Geometry: final body of the model. Coordinates: model frame, mm. Give positions to 0.01 mm unless a question says otherwise; leave off trailing zeros. Write each loop counter-clockwise with the first axis right and the second up, starting at its lowest first coordinate (ties: lowest second). Pieces come first, ordered by that corner, then holes.
Autodesk Inventor part; units mm, degrees
ref_plane "YZ Plane" through (0, 0, 0) normal (1, 0, 0) x (0, 1, 0)
ref_plane "XZ Plane" through (0, 0, 0) normal (0, 1, 0) x (-1, 0, 0)
ref_plane "XY Plane" through (0, 0, 0) normal (0, 0, 1) x (1, 0, 0)
sketch "Sketch1" plane through (0, 0, 0) normal (0, 0, 1) x (1, 0, 0)
  line L0 (-208, 48) -> (208, 48)
  line L1 (208, -48) -> (-208, 48) construction
  line L2 (-208, -48) -> (208, 48) construction
  circle A0 centre (176, 32) radius 4
  circle A1 centre (-176, 32) radius 4
  circle A2 centre (-128, 40) radius 1.85
  circle A3 centre (-133.6569, 37.6569) radius 1.85
  circle A4 centre (-136, 32) radius 1.85
  circle A5 centre (-133.6569, 26.3431) radius 1.85
  circle A6 centre (-128, 24) radius 1.85
  circle A7 centre (-128, 32) radius 4
  circle A8 centre (-122.3431, 26.3431) radius 1.85
  circle A9 centre (-120, 32) radius 1.85
  circle A10 centre (-122.3431, 37.6569) radius 1.85
  circle A11 centre (128, 40) radius 1.85
  circle A12 centre (122.3431, 37.6569) radius 1.85
  circle A13 centre (120, 32) radius 1.85
  circle A14 centre (122.3431, 26.3431) radius 1.85
  circle A15 centre (128, 24) radius 1.85
  circle A16 centre (133.6569, 26.3431) radius 1.85
  circle A17 centre (128, 32) radius 4
  circle A18 centre (136, 32) radius 1.85
  circle A19 centre (133.6569, 37.6569) radius 1.85
  circle A20 centre (104, 32) radius 1.85
  circle A21 centre (88, 32) radius 1.85
  circle A22 centre (72, 32) radius 1.85
  circle A23 centre (56, 32) radius 1.85
  circle A24 centre (40, 32) radius 1.85
  circle A25 centre (24, 32) radius 1.85
  circle A26 centre (8, 32) radius 1.85
  circle A27 centre (-8, 32) radius 1.85
  circle A28 centre (-24, 32) radius 1.85
  circle A29 centre (-40, 32) radius 1.85
  circle A30 centre (-56, 32) radius 1.85
  circle A31 centre (-72, 32) radius 1.85
  circle A32 centre (-88, 32) radius 1.85
  circle A33 centre (-104, 32) radius 1.85
  line L3 (-208, 48) -> (-208, 32)
  line L4 (-128, -48) -> (-208, 32)
  line L5 (208, 48) -> (208, 32)
  line L6 (128, -48) -> (208, 32)
  line L7 (128, -48) -> (-128, -48)
  point P0 (0, 0)
  dimension "d0" = 416
  dimension "d1" = 96
  dimension "d22" = 16
  dimension "d23" = 80
  dimension "d24" = 16
extrude "Extrusion2" add sketch "Sketch1" along normal blind 4
sketch "Sketch2" plane through (0, 0, 0) normal (0, 0, -1) x (-1, 0, 0)
  circle A0 centre (-112, -32) radius 4
  circle A1 centre (112, -32) radius 4
  point P0 (0, 0)
sketch "Sketch3" plane through (0, 0, 0) normal (0, 0, -1) x (-1, 0, 0)
  circle A0 centre (-112, -24) radius 1.85
  circle A1 centre (-104, -32) radius 1.85
  circle A2 centre (-112, -40) radius 1.85
  circle A3 centre (-120, -32) radius 1.85
  circle A4 centre (-112, -8) radius 1.85
  circle A5 centre (112, -8) radius 1.85
  circle A6 centre (120, -32) radius 1.85
  circle A7 centre (112, -40) radius 1.85
  circle A8 centre (104, -32) radius 1.85
  circle A9 centre (112, -24) radius 1.85
  point P0 (0, 0)
hole "Hole1" at (112, -32, 0) at (-112, -32, 0) direction (0, 0, 1) diameter 8 end through all
hole "Hole2" at (-112, -24, 0) at (-112, -8, 0) at (-120, -32, 0) at (-112, -40, 0) at (-104, -32, 0) at (112, -8, 0) at (120, -32, 0) at (112, -40, 0) at (104, -32, 0) at (112, -24, 0) direction (0, 0, 1) diameter 3.7 end through all
properties part number "bot plate"
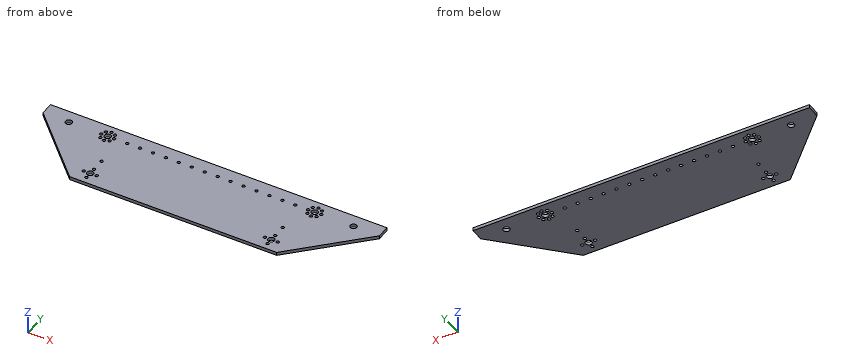
Q1. Section B-B on x = 150. Output: boundary loops of the cut face in (y, z), plus the area to 3 significant figures.
Filled sheet:
outline: (-26, 0) - (48, 0) - (48, 4) - (-26, 4) - close
area: 296 mm2
Q2. Section C-C on z = 2.15. Count the separate pieces of the cut face and the enclosed holes in it, plus the area to 3 significant figures.
Filled sheet:
separate pieces: 1
enclosed holes: 46
area: 32,800 mm2
Q3. Pin query (flat end, axial travel): P1, Ø1.5, axis at x = -161.5, z = 0.5, coming from the -Y side. Return the tip coordinate at first contact, or that it passes through.
Filled sheet:
P1: stops at y = -15.25
Q4. Ray query, line 1 along X through (y, z) = (38, 1); line 2 along Y through (x, z) = (120, 1.25); line 3 along Y through (x, z) = (-112, 1.85). Return the intervals inside material, ascending.
Filled sheet:
line 1: x = -208 to -135.47, -131.84 to -124.16, -120.53 to 120.53, 124.16 to 131.84, 135.47 to 208
line 2: y = -48 to -33.85, -30.15 to 30.15, 33.85 to 48
line 3: y = -48 to -41.85, -38.15 to -36, -28 to -25.85, -22.15 to -9.85, -6.15 to 48
Q5. Section A-A on y = 16. Output: boundary loops of the cut face in (x, z).
Filled sheet:
outline: (-192, 0) - (192, 0) - (192, 4) - (-192, 4) - close
